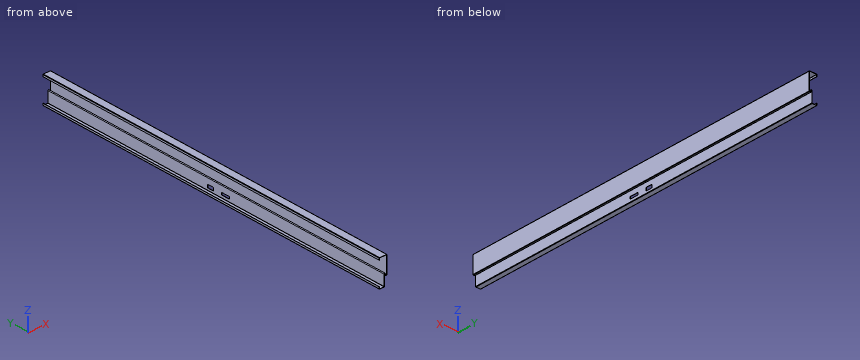
from build123d import *

# Parameters (mm, degrees)
BASE_FLANGE1_DEPTH = 1050
SKETCH2_W          = 18
SKETCH2_H          = 38
SKETCH2_W_2        = 13
SKETCH2_H_2        = 50
CUT_EXTRUDE1_DEPTH = 10


# Sheet-metal steps are written as plain solids
with BuildPart() as part:
    # Sketch1 → Base-Flange1 (new, symmetric)
    with BuildSketch(Plane(origin=(0, 0, 0), x_dir=(1, 0, 0), z_dir=(0, 1, 0))):
        with BuildLine():
            Line((-15, 65), (-15, 74.7634))
            ThreePointArc((-15, 74.7634), (-14.344915027, 76.344915027), (-12.7634, 77))
            Line((-12.7634, 77), (12.7634, 77))
            ThreePointArc((12.7634, 77), (14.344915027, 76.344915027), (15, 74.7634))
            Line((15, 74.7634), (15, 30))
            Line((15, 30), (15, 24))
            Line((15, 24), (15, 13.8))
            ThreePointArc((15, 13.8), (16.769678139, 12.091041686), (18.415834526, 13.91928357))
            Line((18.415834526, 13.91928357), (17.878230266, 21.607382671))
            ThreePointArc((17.878230266, 21.607382671), (18.473636332, 23.288757532), (20.109382021, 24))
            Line((20.109382021, 24), (27.2634, 24))
            ThreePointArc((27.2634, 24), (28.844915027, 23.344915027), (29.5, 21.7634))
            Line((29.5, 21.7634), (29.5, -30))
            Line((29.5, -30), (29.5, -74.7634))
            ThreePointArc((29.5, -74.7634), (28.844915027, -76.344915027), (27.2634, -77))
            Line((27.2634, -77), (15, -77))
            Line((15, -77), (-12.7634, -77))
            ThreePointArc((-12.7634, -77), (-14.344915027, -76.344915027), (-15, -74.7634))
            Line((-15, -74.7634), (-15, -65))
            Line((-15, -65), (-13.5, -65))
            Line((-13.5, -65), (-13.5, -74.7634))
            ThreePointArc((-13.5, -74.7634), (-13.284254855, -75.284254855), (-12.7634, -75.5))
            Line((-12.7634, -75.5), (15, -75.5))
            Line((15, -75.5), (27.2634, -75.5))
            ThreePointArc((27.2634, -75.5), (27.784254855, -75.284254855), (28, -74.7634))
            Line((28, -74.7634), (28, -30))
            Line((28, -30), (28, 21.7634))
            ThreePointArc((28, 21.7634), (27.784254855, 22.284254855), (27.2634, 22.5))
            Line((27.2634, 22.5), (20.109382021, 22.5))
            ThreePointArc((20.109382021, 22.5), (19.570666884, 22.265759992), (19.374576341, 21.712017381))
            Line((19.374576341, 21.712017381), (19.912180601, 14.023918281))
            ThreePointArc((19.912180601, 14.023918281), (16.822027384, 10.591955445), (13.5, 13.8))
            Line((13.5, 13.8), (13.5, 24))
            Line((13.5, 24), (13.5, 30))
            Line((13.5, 30), (13.5, 74.7634))
            ThreePointArc((13.5, 74.7634), (13.284254855, 75.284254855), (12.7634, 75.5))
            Line((12.7634, 75.5), (-12.7634, 75.5))
            ThreePointArc((-12.7634, 75.5), (-13.284254855, 75.284254855), (-13.5, 74.7634))
            Line((-13.5, 74.7634), (-13.5, 65))
            Line((-13.5, 65), (-15, 65))
        make_face()
    extrude(amount=BASE_FLANGE1_DEPTH, both=True)

    # Sketch2 → Cut-Extrude1 (cut)
    with BuildSketch(Plane(origin=(15, 0, 0), x_dir=(0, 0, -1), z_dir=(1, 0, 0))):
        with Locations((54.5, 34)):
            Rectangle(SKETCH2_W, SKETCH2_H)
        with Locations((54.5, -59)):
            Rectangle(SKETCH2_W_2, SKETCH2_H_2)
    extrude(amount=-CUT_EXTRUDE1_DEPTH, mode=Mode.SUBTRACT)


solid = part.part
Read the model definition and answer for the solid it produces. Units are mm, in the model's axes. Coordinates: 2 decimals unless noted, no trailing zeros. Loops run counter-clockwise (first coordinate to the right, second up) from the corner with the lowest first, then second, coordinate; pieces in that order, holes last.
Q1. Each of these flat-tipped pins is pushed along its axis until it touches: pin 1 Ø5 at (y, z) = (627.5, -33.5) entering from -X; pin 2 Ø1 at (y, z) = (537.5, -44) entering from +X; pin 3 Ø1 at (y, z) = (-69, 32.5) entering from -X. Where does it stop, or does it pass through?
Q2. Consider probe 1 along X at (y, z) = (150.5, 70); probe 2 along Z at (x, y) = (-3.5, -421); probe 3 along Z at (x, y) = (22, -466). Determine where each line is inside the solid, lowest interval first.
Q3. The part is cut by section C-C on z = 35.5. Write down the section's boundary in (x, y), and give its area (3 significant figures).
Q4. The part is cut by section A-A on x = -5. Write down the section's boundary in (y, z).
Results below:
1. pin 1: stops at x = 13.5
1. pin 2: stops at x = 15
1. pin 3: stops at x = 28
2. probe 1: x = -15 to -13.5, 28 to 29.5
2. probe 2: z = -77 to -75.5, 75.5 to 77
2. probe 3: z = -24 to -22.5, 75.5 to 77
3. outline: (28, -1050) - (29.5, -1050) - (29.5, 1050) - (28, 1050) - close
3. area: 3,150 mm2
4. outline: (-1050, -77) - (1050, -77) - (1050, -75.5) - (-1050, -75.5) - close; (-1050, 75.5) - (1050, 75.5) - (1050, 77) - (-1050, 77) - close
